Read the model definition and answer for the solid it produces. Units are mm, in the model's axes. Face numbers are marked on the shaded views. A direction names the side the tool comes from. Coordinates: 2 decimals unless noted, no trailing zeros. Write each loop counter-clockwise with the first axis right and the second up, starting at its lowest first coordinate (ties: lowest second). Pieces come first, ordered by that corner, then holes. Notation, with made-up numbers: (66, 6) -> (107, 6) arc R18 ccw to (107, 14) -> close; hole circle Ø8 at (34.5, -30.75). An arc over 180 degrees is marked (long way). Write item = value, one per line. Start each with the question number.
1) Find the intervals of material crossed by line 1 along X through (y, z) = (11.5, 1.25); line 2 along Y through (x, z) = (10, 1.05); line 3 along Z through (x, y) = (14.25, 8), in increasing order. Write a range as from..to.
2) Section B-B (x = 10) is taken. Determine the outline of the cut face in (y, z), plus the area to 3 significant figures.
3) Flat-ended cylindrical pins translate along their axes: pin 1 Ø6.5 at (x, y) = (7, 15.5) entering from +Z; pin 2 Ø8 at (x, z) = (11.5, 13) entering from +Y; pin 3 Ø10.5 at (x, z) = (10, 11.5) entering from +Y. Find the tip coordinate at first contact, or state that the pin passes through.
4) For a pull along Y with two mould halves and no side action, classify the marked faces 3, 4, 5 and 6 as released by +Y, released by -Y, zero draft, split by the parting line, or undercut.
5) Section C-C (x = 4.5) is taken. Determine the outline of the cut face in (y, z).
6) Section A-A (y = 11.5) is taken. Determine the outline of the cut face in (x, z), plus the area to 3 significant figures.
7) Section D-D (z = 16.5) is taken. Determine the outline of the cut face in (x, y), plus the area to 3 significant figures.
8) A tool of negligible diameter and unlimited length cuts with its end or side. For the marked faces 1 and 2, from which of +Z, -Z, +X, -X, +Y, -Y can it reach the whole face along a straight path? Write none if from no direction.
Autodesk Fusion 360 part; units mm, degrees
sketch "Sketch1" plane through (0, 0, 0) normal (0, 0, 1) x (1, 0, 0)
  line L0 (0, 0) -> (20, 0)
  line L1 (20, 0) -> (20, 20)
  line L2 (20, 20) -> (0, 20)
  line L3 (0, 20) -> (0, 0)
  dimension "d1" = 20
  dimension "d2" = 20
extrude "Extrude1" add sketch "Sketch1" along normal blind 3
sketch "Sketch2" plane through (0, 0, 3) normal (0, 0, 1) x (-1, 0, 0)
  line L0 (0, -20) -> (0, 0)
  line L1 (0, 0) -> (-20, 0)
  line L2 (-20, 0) -> (-20, -20)
  line L3 (-20, -20) -> (0, -20)
  line L4 (0, 0) -> (-20, 0)
  line L5 (-20, 0) -> (-20, -3)
  line L6 (-20, -3) -> (0, -3)
  line L7 (0, -3) -> (0, 0)
  dimension "d5" = 20
  dimension "d6" = 3
extrude "Extrude2" add sketch "Sketch2" along normal blind 17 contours L0 L1 L2 L4 L5 L6 L7
sketch "Sketch3" plane through (0, 0, 3) normal (0, 0, 1) x (-1, 0, 0)
  line L0 (0, -3) -> (-20, -3)
  line L1 (-20, -3) -> (-20, -20)
  line L2 (-20, -20) -> (0, -20)
  line L3 (0, -20) -> (0, -3)
  line L4 (-10, -20) -> (-10, -3) construction
  point P0 (-10, -11.5)
hole "Hole1" at (10, 11.5, 3) direction (0, 0, -1) diameter 3.4 depth 10 tip angle 180 countersink diameter 6.3 countersink angle 90
fillet "Fillet1" radius 4 1 edges at (10, 3, 3)
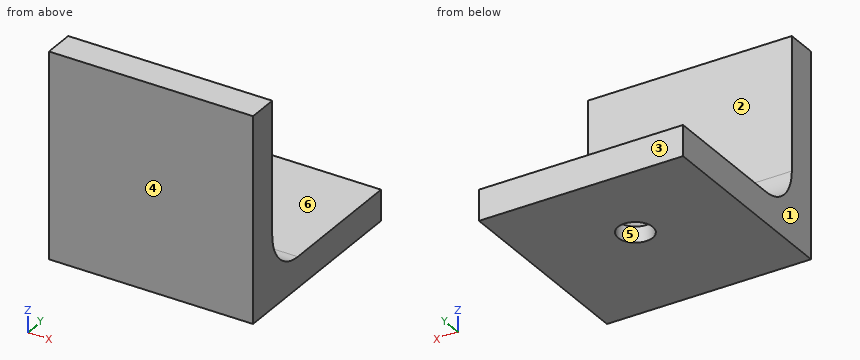
Answer key:
q1.line_1 = 0..8.3, 11.7..20
q1.line_2 = 0..9.8, 13.2..20
q1.line_3 = 0..3
q2.outline = (0, 0) -> (9.8, 0) -> (9.8, 1.55) -> (8.35, 3) -> (7, 3) arc R4 cw to (3, 7) -> (3, 20) -> (0, 20) -> close; (13.2, 0) -> (20, 0) -> (20, 3) -> (14.65, 3) -> (13.2, 1.55) -> close
q2.area = 102 mm^2
q3.pin_1 = 3
q3.pin_2 = 3
q3.pin_3 = 3.07
q4.face_3 = released by +Y
q4.face_4 = released by -Y
q4.face_5 = undercut
q4.face_6 = zero draft
q5.outline = (0, 0) -> (20, 0) -> (20, 3) -> (7, 3) arc R4 cw to (3, 7) -> (3, 20) -> (0, 20) -> close
q6.outline = (0, 0) -> (8.3, 0) -> (8.3, 1.55) -> (6.85, 3) -> (0, 3) -> close; (11.7, 0) -> (20, 0) -> (20, 3) -> (13.15, 3) -> (11.7, 1.55) -> close
q6.area = 47.7 mm^2
q7.outline = (0, 0) -> (20, 0) -> (20, 3) -> (0, 3) -> close
q7.area = 60.0 mm^2
q8.face_1 = +Z, -Z, -X, +Y, -Y
q8.face_2 = +Z, +X, -X, +Y
